```python
from build123d import *

# Parameters (mm, degrees)
SKETCH1_W               = 56.4
SKETCH1_H               = 56.4
BOSS_EXTRUDE1_DEPTH     = 20
SKETCH2_R               = 20.904355549
CUT_EXTRUDE2_DEPTH      = 20
SKETCH3_W               = 56.4
SKETCH3_H               = 34.3
BOSS_EXTRUDE2_DEPTH     = 20
FILLET1_R               = 3
TAP_DRILL_FOR_M6_TAP1_D = 5
M6_CLEARANCE_HOLE1_D    = 6.6


with BuildPart() as part:
    # Sketch1 → Boss-Extrude1 (new body)
    with BuildSketch(Plane.XY):
        with Locations((0, 25)):
            Rectangle(SKETCH1_W, SKETCH1_H)
    extrude(amount=BOSS_EXTRUDE1_DEPTH)

    # Sketch2 → Cut-Extrude2 (cut)
    with BuildSketch(Plane.XY.offset(20)):
        with Locations((0, 25)):
            Circle(SKETCH2_R)
    extrude(amount=-CUT_EXTRUDE2_DEPTH, mode=Mode.SUBTRACT)

    # Sketch3 → Boss-Extrude2 (add)
    with BuildSketch(Plane(origin=(0, 0, 0), x_dir=(-1, 0, 0), z_dir=(0, 0, -1))):
        with Locations((0, -20.35)):
            Rectangle(SKETCH3_W, SKETCH3_H)
    extrude(amount=-BOSS_EXTRUDE2_DEPTH)

    # Fillet1
    fillet1_edges = [part.edges().sort_by_distance(p)[0] for p in [
        (28.2, -37.5, 10),
        (-28.2, -37.5, 10),
        (28.2, 53.2, 10),
        (-28.2, 53.2, 10),
    ]]
    fillet(fillet1_edges, radius=FILLET1_R)

    # Tap Drill for M6 Tap1 (through all)
    with Locations(Plane(origin=(0, 0, 0), x_dir=(-1, 0, 0), z_dir=(0, 0, -1))):
        with Locations((-23.57, 48.57), (23.57, 48.57), (-23.57, 1.43), (23.57, 1.43)):
            Hole(TAP_DRILL_FOR_M6_TAP1_D / 2)

    # M6 Clearance Hole1 (through all)
    with Locations(Plane(origin=(0, 0, 0), x_dir=(-1, 0, 0), z_dir=(0, 0, -1))):
        with Locations((-20, -7.5), (-20, -27.5), (20, -28.237657735), (20, -7.5)):
            Hole(M6_CLEARANCE_HOLE1_D / 2)


solid = part.part
```
Work out the finished part from the listing and answer in its coordinate system (mm). Give positions to 0.01 mm unless a question says otherwise; leave off trailing zeros. Loops run counter-clockwise (first coordinate to the right, second up) from the corner with the lowest first, then second, coordinate; pieces in that order, holes last. Notation, with made-up numbers: M -17.75,-38 L 12.25,-38 A24 cw 12.25,1 Z; hole C 87,4 d10. An arc over 180 degrees is marked long. One line per item, written item: value. Start each with the question number.
1. Find section C-C (z = 10.25). State how many separate pieces and enclosed holes the cut face has, and give its area (3 significant figures).
2. Find section A-A (y = -7.5). Give the vertices of the cut face in (x, z), and give its area (3 significant figures).
3. Find section B-B (y = 43). Give the vertices of the cut face in (x, z).
4. Find section D-D (x = -6). Give the vertices of the cut face in (y, z).
5. Determine the mould class of faces 1 (the face through (21.774, -24.717, 10.14)), 2 (the face through (27.34, -36.6, 10.14)), 3 (the face through (0, -37.5, 10)) for opening direction X: released by +X, released by -X, zero draft, split by the parting line, or undercut.
6. Find the intervals of material crossed by probe 1 along Y at (x, z) = (23.57, 8.5); probe 2 along X at (y, z) = (-25.5, 9.5); probe 3 along Y at (x, z) = (18, 11.75), in increasing order.
Reported:
1. separate pieces: 1
1. enclosed holes: 9
1. area: 3,520 mm²
2. outline: M -28.2,0 L -23.3,0 L -23.3,20 L -28.2,20 Z; M -16.7,0 L 16.7,0 L 16.7,20 L -16.7,20 Z; M 23.3,0 L 28.2,0 L 28.2,20 L 23.3,20 Z
2. area: 864 mm²
3. outline: M -28.2,0 L -10.63,0 L -10.63,20 L -28.2,20 Z; M 10.63,0 L 28.2,0 L 28.2,20 L 10.63,20 Z
4. outline: M -37.5,0 L 4.98,0 L 4.98,20 L -37.5,20 Z; M 45.02,0 L 53.2,0 L 53.2,20 L 45.02,20 Z
5. face 1: undercut
5. face 2: released by +X
5. face 3: zero draft
6. probe 1: y = -37.5 to -1.07, 3.93 to 46.07, 51.07 to 53.2
6. probe 2: x = -28.2 to -21.84, -18.16 to 17.38, 22.62 to 28.2
6. probe 3: y = -37.5 to -30.12, -24.88 to -10.12, -4.88 to 14.37, 35.63 to 53.2
